Part model, mm, in its own coordinate system. A direction names the side the tool comes from. Round coordinates to 2 decimals unless told otherwise and drop trailing zeros. Write each loop counter-clockwise with the first axis right and the second up, starting at its lowest first coordinate (ties: lowest second). Pieces come first, ordered by that corner, then holes. Notation, with made-up numbers: (5, -27) -> (21, -27) arc R34 cw to (21, 12) -> close; hole circle Ø8 at (24.25, 39.25). An arc over 180 degrees is marked (long way). Return JSON: item names as keys, results as strings. Group by question number.
(1) Tool access for faces 4 (the cylindrical face through (6, 11, 11)), 5 (the cylindrical face through (10.4, 2.93, 2.46)), 6 (the cylindrical face through (7.899, 9.074, 3.698)): list every direction of +Z, -Z, +X, -X, +Y, -Y with a clear straight run to the whole face (end or side of a thin tool).
(2) Saw through at A-A (x = 4). List the corners of the cut face in (y, z).
(3) Saw through at D-D (x = 42.5). List the corners of the cut face in (y, z), plus the area to 3 significant figures.
(4) Saw through at B-B (z = 11). List the corners of the cut face in (x, y), plus the area to 3 significant figures.
(5) Drop flat-ended pins along their axis: pin 1 Ø1.7 at (x, y) = (9, 11.5) entering from -Z; pin 2 Ø5 at (x, y) = (27, 10) entering from +Z; pin 3 Ø1 at (y, z) = (8, 6) entering from -X. Give the stop position or say it passes through.
(6) Mould opens along Y. For faces 1 (the flat face through (31, 17, 2)), 2 (the cylindrical face through (54.718, 10.144, 3.698)), 3 (the flat face through (0, 8, 2)) say: +Y half, -Y half, draft (parallel to the pull), parting line (faces both ways), or undercut.
(7) Saw through at C-C (y = 11). State how many separate pieces and enclosed holes the cut face has, plus the area to 3 significant figures.
(8) Drill centre lines: L1, parallel to Y at x = 57.1, z = 2.9; L2, parallel to X at y = 14.1, z = 2.05; L3, parallel to Y at x = 52, z = 3. Where is each one in solid material? Low to high. Write a range as from..to.
from build123d import *

# Parameters (mm, degrees)
F0_W      = 62
F0_H      = 17
F1_DEPTH  = 5
F2_R      = 5
F3_DEPTH  = 1
F4_R      = 4
F5_DEPTH  = 11
F6_R      = 2.85
F7_DEPTH  = 7.5
F8_R      = 1.6
F9_DEPTH  = 25
F10_R     = 1.5
F11_DEPTH = 5


with BuildPart() as f1:
    # F0 (on Top) → F1 (new body)
    with BuildSketch(Plane.XY):
        with Locations((31, 8.5)):
            Rectangle(F0_W, F0_H)
    extrude(amount=F1_DEPTH)

    # F2 (on face) → F3 (join)
    with BuildSketch(Plane.XY.offset(5)):
        with Locations((10, 11)):
            Circle(F2_R)
        with Locations((52, 11)):
            Circle(F2_R)
    extrude(amount=F3_DEPTH)

    # F4 (on face) → F5 (join)
    with BuildSketch(Plane.XY.offset(6)):
        with Locations((52, 11)):
            Circle(F4_R)
        with Locations((10, 11)):
            Circle(F4_R)
    extrude(amount=F5_DEPTH)

    # F6 (on face) → F7 (cut)
    with BuildSketch(Plane(origin=(0, 0, 0), x_dir=(1, 0, 0), z_dir=(0, 0, -1))):
        with Locations((52, -11)):
            Circle(F6_R)
        with Locations((10, -11)):
            Circle(F6_R)
    extrude(amount=-F7_DEPTH, mode=Mode.SUBTRACT)

    # F8 (on face) → F9 (cut)
    with BuildSketch(Plane.XY.offset(17)):
        with Locations((52, 11)):
            Circle(F8_R)
        with Locations((10, 11)):
            Circle(F8_R)
    extrude(amount=-F9_DEPTH, mode=Mode.SUBTRACT)

    # F10 (on face) → F11 (cut, through all)
    with BuildSketch(Plane(origin=(0, 0, 0), x_dir=(1, 0, 0), z_dir=(0, 0, -1))):
        with Locations((57.1, -14.1)):
            Circle(F10_R)
        with Locations((50.1, -3)):
            Circle(F10_R)
        with Locations((11.9, -3)):
            Circle(F10_R)
        with Locations((4.9, -14.1)):
            Circle(F10_R)
        with Locations((57.1, -3)):
            Circle(F10_R)
        with Locations((4.9, -3)):
            Circle(F10_R)
    extrude(amount=-F11_DEPTH, mode=Mode.SUBTRACT)


solid = f1.part
Computed values:
{
 "1": {"face 4": "+Z", "face 5": "+Z, -Z", "face 6": "-Z"},
 "2": {"outline": "(0, 0) -> (1.8, 0) -> (1.8, 5) -> (0, 5) -> close; (4.2, 0) -> (12.9, 0) -> (12.9, 5) -> (4.2, 5) -> close; (15.3, 0) -> (17, 0) -> (17, 5) -> (15.3, 5) -> close"},
 "3": {"outline": "(0, 0) -> (17, 0) -> (17, 5) -> (0, 5) -> close", "area": "85.0 mm2"},
 "4": {"outline": "circle Ø8 at (10, 11); circle Ø8 at (52, 11); hole circle Ø3.2 at (10, 11); hole circle Ø3.2 at (52, 11)", "area": "84.4 mm2"},
 "5": {"pin 1": "z = 7.5", "pin 2": "z = 5", "pin 3": "x = 5.67"},
 "6": {"face 1": "+Y half", "face 2": "undercut", "face 3": "draft"},
 "7": {"separate pieces": "3", "enclosed holes": "0", "area": "360 mm2"},
 "8": {"L1": "0..1.5, 4.5..12.6, 15.6..17", "L2": "0..3.4, 6.4..55.6, 58.6..62", "L3": "0..8.15, 13.85..17"}
}
